```python
from build123d import *

# Parameters (mm, degrees)
SKETCH_1_W          = 63
SKETCH_1_H          = 10
EXTRUDE_1_DEPTH     = 2
SKETCH_4_W          = 2
SKETCH_4_H          = 10
EXTRUDE_2_DEPTH     = 93
SKETCH_5_W          = 61
SKETCH_5_H          = 10
EXTRUDE_3_DEPTH     = 1
SKETCH_6_W          = 10
SKETCH_6_H          = 92
EXTRUDE_4_DEPTH     = 1
SKETCH_7_W          = 3
SKETCH_7_H          = 10
EXTRUDE_5_DEPTH     = 93
SKETCH_10_W         = 26.594312394
SKETCH_10_H         = 101.559656513
CUT_EXTRUDE_1_DEPTH = 93


with BuildPart() as part:
    # 草图1 → 凸台-拉伸1 (new body)
    with BuildSketch(Plane(origin=(0, 0, 0), x_dir=(1, 0, 0), z_dir=(0, 1, 0))):
        Rectangle(SKETCH_1_W, SKETCH_1_H)
    extrude(amount=EXTRUDE_1_DEPTH)

    # 草图4 → 凸台-拉伸2 (add)
    with BuildSketch(Plane(origin=(0, 2, 0), x_dir=(1, 0, 0), z_dir=(0, 1, 0))):
        with Locations((30.5, 0)):
            Rectangle(SKETCH_4_W, SKETCH_4_H)
    extrude(amount=EXTRUDE_2_DEPTH)

    # 草图5 → 凸台-拉伸3 (add)
    with BuildSketch(Plane(origin=(0, 2, 0), x_dir=(1, 0, 0), z_dir=(0, 1, 0))):
        with Locations((-1, 0)):
            Rectangle(SKETCH_5_W, SKETCH_5_H)
    extrude(amount=EXTRUDE_3_DEPTH)

    # 草图6 → 凸台-拉伸4 (add)
    with BuildSketch(Plane.ZY.offset(-29.5)):
        with Locations((0, 49)):
            Rectangle(SKETCH_6_W, SKETCH_6_H)
    extrude(amount=EXTRUDE_4_DEPTH)

    # 草图7 → 凸台-拉伸5 (add)
    with BuildSketch(Plane(origin=(0, 0, -5), x_dir=(-1, 0, 0), z_dir=(0, 0, -1))):
        with Locations((-30, 5)):
            Rectangle(SKETCH_7_W, SKETCH_7_H)
    extrude(amount=EXTRUDE_5_DEPTH)

    # 草图10 → 切除-拉伸1 (cut)
    with BuildSketch(Plane.ZY.offset(-28.5)):
        with Locations((8.297156197, 60.779828257)):
            Rectangle(SKETCH_10_W, SKETCH_10_H)
    extrude(amount=-CUT_EXTRUDE_1_DEPTH, mode=Mode.SUBTRACT)


solid = part.part
```
Check sheet for the modelled part. Datum: model origin and axes. Units: mm. A direction names the side the tool comes from. Give positions to 0.01 mm unless a question says otherwise; leave off trailing zeros. Order: outer loops, then holes, each group sorted by start corner. A loop starts at its lowest first (then second) coordinate and runs counter-clockwise, first axis right, second up. Notation, with made-up numbers: M -14,-16.5 L 26,-16.5 A25 ccw 26,8.5 Z; hole C 32.25,-16.5 d11. An arc over 180 degrees is marked long. Answer in a Markdown table with one row per item.
1) Access from +Z, -Z, +X, -X, +Y, -Y to the whole of each face (thin tool, end or side, straight path). Record for faces 1 (the flat face through (-1, 1, -5)), 2 (the flat face through (30, 5, -98)), 3 (the flat face through (-2, 3, 0)).
Filled sheet:
| item | result |
|---|---|
| face 1 | -Z, -X, +Y, -Y |
| face 2 | -Z, +X, -X, +Y, -Y |
| face 3 | +Z, -Z, -X, +Y |
2) Cross-section at D-D, the plane z = -12. Enter the section's corners in (x, y), plus the area to 3 significant figures.
Filled sheet:
| item | result |
|---|---|
| outline | M 28.5,0 L 31.5,0 L 31.5,10 L 28.5,10 Z |
| area | 30.0 mm2 |
3) Gauge pin test, flat ends, axial feed: P1, Ø11, axis at x = 0, z = -2, coming from the +Y side; P2, Ø0.9, axis at x = 4.5, y = 1, coming from the -Z side. Record the tip position at first contact, or that the pin passes through.
Filled sheet:
| item | result |
|---|---|
| P1 | stops at y = 3 |
| P2 | stops at z = -5 |
4) Cross-section at A-A, the plane z = -0.5. Enter the section's corners in (x, y), plus the area to 3 significant figures.
Filled sheet:
| item | result |
|---|---|
| outline | M -31.5,0 L 31.5,0 L 31.5,10 L 28.5,10 L 28.5,3 L -31.5,3 Z |
| area | 210 mm2 |
5) Cross-section at B-B, the plane y = 1.5. Enter the section's corners in (x, z), plus the area to 3 significant figures.
Filled sheet:
| item | result |
|---|---|
| outline | M -31.5,-5 L 28.5,-5 L 28.5,-98 L 31.5,-98 L 31.5,5 L -31.5,5 Z |
| area | 909 mm2 |
6) Cross-section at C-C, the plane x = -12. Enter the section's corners in (y, z).
Filled sheet:
| item | result |
|---|---|
| outline | M 0,-5 L 3,-5 L 3,5 L 0,5 Z |
7) Thickness scan on L1, parallel to X at y = 5.5, z = -27.5; L2, parallel to Z at x = -14.5, y = 2. Record the ranges inside material, lowest first. Write a range as [from, to].
Filled sheet:
| item | result |
|---|---|
| L1 | x = [28.5, 31.5] |
| L2 | z = [-5, 5] |
